The model under review builds one solid part; all positions refer to its coordinate system, in mm. A direction names the side the tool comes from. Round coordinates to 2 decimals unless told otherwise and drop trailing zeros. Loops run counter-clockwise (first coordinate to the right, second up) from the corner with the lowest first, then second, coordinate; pieces in that order, holes last. Notation, with made-up numbers: (55, -7.5) -> (71, -7.5) arc R28 cw to (71, 30.5) -> close; hole circle Ø1 at (16.5, 62.25). An arc over 180 degrees is marked (long way). Write each question's results on one line, items separated by ' | '. Start each with the question number.
Item 1: We need section A-A (x = 24.5). Give the boundary of the cut face in (y, z) (3 decimals).
Item 2: Clearance check with flat-ended pins moving along their axes: pin 1 Ø4.5 at (x, y) = (-31.5, 7.5) entering from +Z (3 decimals); pin 2 Ø8 at (y, z) = (10, 0.5) entering from -X; pin 3 Ø2.5 at (x, y) = (-32.5, 4.5) entering from -Z (3 decimals); pin 4 Ø2.5 at (x, z) = (24.5, 24.455) entering from -Y. State where each tip first meets the part, or that it passes through.
Item 3: Tool access review of faces 1 (the flat face through (32, 8, -19.905)), 2 (the flat face through (-27.7, 8, 21)), 3 (the flat face through (27.7, 8, 9)): name each direction out of +Z, -Z, +X, -X, +Y, -Y from which nothing blocks a thin tool from reaching the whole face with its end or side.
Item 4: Mouldability with a two-part tool opening along Z and no side actions: class faces 4 (the flat face through (-32, 8, -5.305)), 5 (the cylindrical face through (24.29, 7.89, 22.87)), 6 (the flat face through (0, 8, -27.655)), 7 (the flat face through (36.2, 8, -15)) as pulls with the +Z half, pulls with the -Z half, needs draft (parallel to the pull), parting line crosses it, or undercut.
Item 5: For L1, parallel to Z at x = 24.5, y = 9.5 (3 decimals); L2, parallel to X at y = 11, z = 23; L3, parallel to X at y = 3, z = -8, list the stretches that pass through material, from the lowest coordinate up. Write a range as from..to.
Item 6: We need section B-B (y = 9). Give the boundary of the cut face in (x, z) (3 decimals).
Item 7: We need section C-C (z = 14). Give the boundary of the cut face in (x, y).
from build123d import *

# Parameters (mm, degrees)
SKETCH1_R           = 1.6
BOSS_EXTRUDE1_DEPTH = 16


with BuildPart() as part:
    # Sketch1 → Boss-Extrude1 (new body)
    with BuildSketch(Plane(origin=(0, 0, 0), x_dir=(1, 0, 0), z_dir=(0, 1, 0))):
        Polygon((-27.7, 27.655), (27.7, 27.655), (27.7, 19.905), (36.2, 19.905), (36.2, 9.705), (27.7, 9.705), (27.7, -27.655), (-27.7, -27.655), (-27.7, -15.095), (-36.2, -15.095), (-36.2, -4.895), (-27.7, -4.895), (-27.7, 5.305), (-36.2, 5.305), (-36.2, 15.505), (-27.7, 15.505), align=None)
        with Locations((-24.5, 24.455)):
            Circle(SKETCH1_R, mode=Mode.SUBTRACT)
        with Locations((24.5, 24.455)):
            Circle(SKETCH1_R, mode=Mode.SUBTRACT)
        with Locations((-24.5, -24.455)):
            Circle(SKETCH1_R, mode=Mode.SUBTRACT)
        with Locations((24.5, -24.455)):
            Circle(SKETCH1_R, mode=Mode.SUBTRACT)
    extrude(amount=BOSS_EXTRUDE1_DEPTH)


solid = part.part
Here are the results:
1) outline: (0, -27.655) -> (16, -27.655) -> (16, -26.055) -> (0, -26.055) -> close; (0, -22.855) -> (16, -22.855) -> (16, 22.855) -> (0, 22.855) -> close; (0, 26.055) -> (16, 26.055) -> (16, 27.655) -> (0, 27.655) -> close
2) pin 1: stops at z = 15.095 | pin 2: stops at x = -27.7 | pin 3: stops at z = -15.505 | pin 4: passes through
3) face 1: -Z, +X, +Y, -Y | face 2: +Z, -X, +Y, -Y | face 3: +Z, +X, +Y, -Y
4) face 4: undercut | face 5: undercut | face 6: pulls with the -Z half | face 7: needs draft
5) L1: z = -27.655..-26.055, -22.855..22.855, 26.055..27.655 | L2: x = -27.7..-25.17, -23.83..23.83, 25.17..27.7 | L3: x = -36.2..27.7
6) outline: (-36.2, -15.505) -> (-27.7, -15.505) -> (-27.7, -27.655) -> (27.7, -27.655) -> (27.7, -19.905) -> (36.2, -19.905) -> (36.2, -9.705) -> (27.7, -9.705) -> (27.7, 27.655) -> (-27.7, 27.655) -> (-27.7, 15.095) -> (-36.2, 15.095) -> (-36.2, 4.895) -> (-27.7, 4.895) -> (-27.7, -5.305) -> (-36.2, -5.305) -> close; hole circle Ø3.2 at (-24.5, -24.455); hole circle Ø3.2 at (-24.5, 24.455); hole circle Ø3.2 at (24.5, -24.455); hole circle Ø3.2 at (24.5, 24.455)
7) outline: (-36.2, 0) -> (27.7, 0) -> (27.7, 16) -> (-36.2, 16) -> close
